Study the drawing (mm; zero at the part's minimum x, y, z) and answer. Coordinates: 2 decimals unless noted, no trailing zeros. Loops run counter-clockwise (first coordinate to the right, second up) from the corner with the lowest first, then second, coordinate; pieces in that order, holes last. Notation, with made-up numbers: (2, 89) - (39, 89) arc R17 cw to (39, 100) - close; hole circle Ø4 at (18.25, 36.25). An arc over 180 degrees is marked (long way). One line per item, written item: value. Start each with the question number.
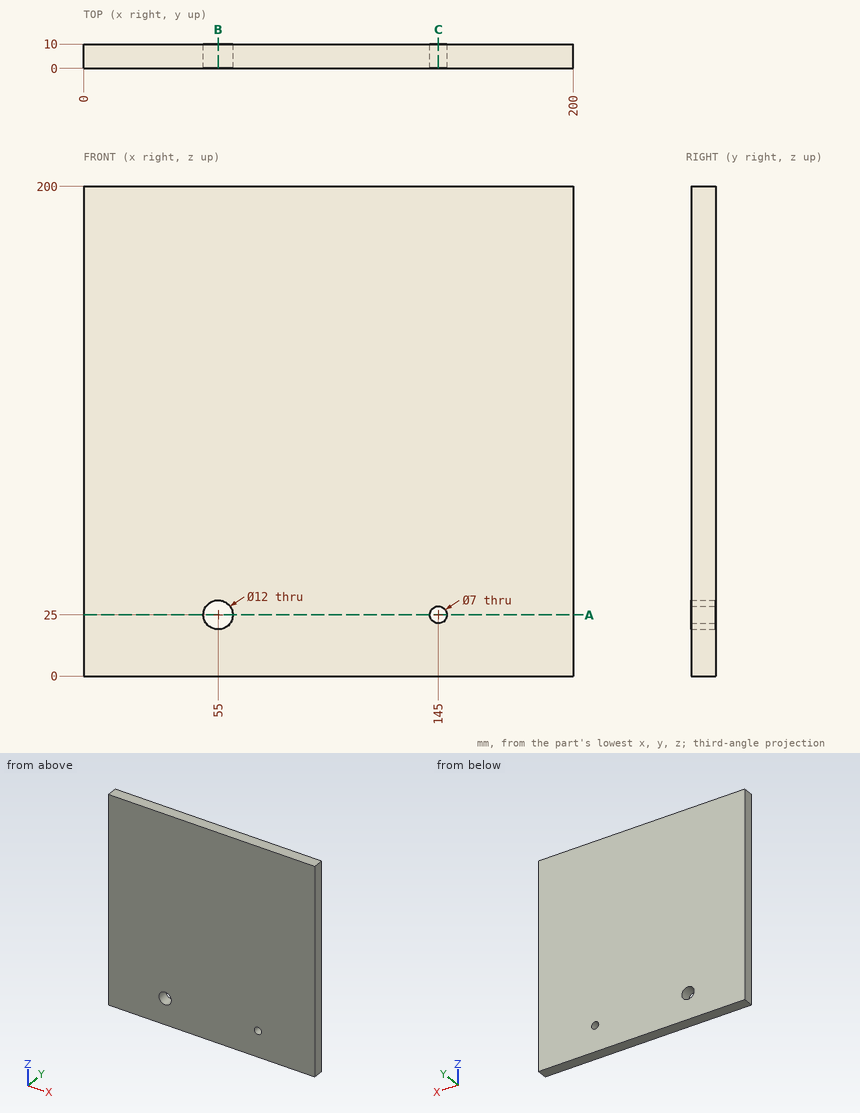
1) Section A-A, the plane z = 25 is taken. Determine the outline of the cut face in (x, y).
2) Section C-C, the plane x = 145 is taken. Determine the outline of the cut face in (y, z), and give its area (3 significant figures).
3) Straight lines are drawn through the part: L1, parallel to X at y = 5.5, z = 25; L2, parallel to Z at x = 55, y = 2.75; L3, parallel to X at y = 5.5, z = 20. For each, find the intervals that lie inside material, in ascending order.
4) Section B-B, the plane x = 55 is taken. Determine the outline of the cut face in (y, z), and give its area (3 significant figures).
Answer below:
1. outline: (0, 0) - (49, 0) - (49, 10) - (0, 10) - close; (61, 0) - (141.5, 0) - (141.5, 10) - (61, 10) - close; (148.5, 0) - (200, 0) - (200, 10) - (148.5, 10) - close
2. outline: (0, 0) - (10, 0) - (10, 21.5) - (0, 21.5) - close; (0, 28.5) - (10, 28.5) - (10, 200) - (0, 200) - close
2. area: 1,930 mm2
3. L1: 0 to 49, 61 to 141.5, 148.5 to 200
3. L2: 0 to 19, 31 to 200
3. L3: 0 to 51.68, 58.32 to 200
4. outline: (0, 0) - (10, 0) - (10, 19) - (0, 19) - close; (0, 31) - (10, 31) - (10, 200) - (0, 200) - close
4. area: 1,880 mm2
